Build history of the part. All positions in model axes, mm. Face numbers are marked on the shaded views. A direction names the side the tool comes from. Round coordinates to 2 decimals unless told otherwise and drop trailing zeros. Write each loop counter-clockwise with the first axis right and the second up, starting at its lowest first coordinate (ties: lowest second). Pieces come first, ordered by that corner, then holes.
from build123d import *

# Parameters (mm, degrees)
SKETCH2_R           = 1.315325132
SKETCH2_R_2         = 1.3
BOSS_EXTRUDE1_DEPTH = 3
CUT_EXTRUDE1_DEPTH  = 10
BOSS_EXTRUDE3_DEPTH = 15
SKETCH6_R           = 2.2
CUT_EXTRUDE2_DEPTH  = 10


with BuildPart() as part:
    # Sketch2 → Boss-Extrude1 (new body)
    with BuildSketch(Plane.XZ):
        with BuildLine():
            Line((-23.009319596, 31.276283835), (22.990680404, 31.490636875))
            ThreePointArc((22.990680404, 31.490636875), (24.41091474, 30.908163296), (25, 29.490658589))
            Line((25, 29.490658589), (25, -4.5))
            ThreePointArc((25, -4.5), (25.585786438, -5.914213562), (27, -6.5))
            Line((27, -6.5), (38, -6.5))
            ThreePointArc((38, -6.5), (39.414213562, -7.085786438), (40, -8.5))
            Line((40, -8.5), (40, -34.5))
            ThreePointArc((40, -34.5), (39.414213562, -35.914213562), (38, -36.5))
            Line((38, -36.5), (-38, -36.5))
            ThreePointArc((-38, -36.5), (-39.414213562, -35.914213562), (-40, -34.5))
            Line((-40, -34.5), (-40, -8.5))
            ThreePointArc((-40, -8.5), (-39.414213562, -7.085786438), (-38, -6.5))
            Line((-38, -6.5), (-27, -6.5))
            ThreePointArc((-27, -6.5), (-25.585786438, -5.914213562), (-25, -4.5))
            Line((-25, -4.5), (-25, 29.276305549))
            ThreePointArc((-25, 29.276305549), (-24.417504708, 30.687220289), (-23.009319596, 31.276283835))
        make_face()
        with Locations(Location((22.009080877, 28.712344932, 0), (0, 0, 270))):
            Circle(SKETCH2_R, mode=Mode.SUBTRACT)
        with Locations(Location((-22, 28.7, 0), (0, 0, 270))):
            Circle(SKETCH2_R_2, mode=Mode.SUBTRACT)
        with Locations(Location((-33.75, -27.3, 0), (0, 0, 270))):
            Circle(SKETCH2_R_2, mode=Mode.SUBTRACT)
        with Locations(Location((33.75, -27.3, 0), (0, 0, 270))):
            Circle(SKETCH2_R_2, mode=Mode.SUBTRACT)
    extrude(amount=BOSS_EXTRUDE1_DEPTH)

    # Sketch3 → Cut-Extrude1 (cut)
    with BuildSketch(Plane.XZ.offset(3)):
        with BuildLine():
            Line((-18, 26.233664787), (18, 26.233664787))
            ThreePointArc((18, 26.233664787), (19.414213562, 25.64787835), (20, 24.233664787))
            Line((20, 24.233664787), (20, -14.643421245))
            ThreePointArc((20, -14.643421245), (19.414213562, -16.057634807), (18, -16.643421245))
            Line((18, -16.643421245), (-18, -16.643421245))
            ThreePointArc((-18, -16.643421245), (-19.414213562, -16.057634807), (-20, -14.643421245))
            Line((-20, -14.643421245), (-20, 24.233664787))
            ThreePointArc((-20, 24.233664787), (-19.414213562, 25.64787835), (-18, 26.233664787))
        make_face()
    extrude(amount=-CUT_EXTRUDE1_DEPTH, mode=Mode.SUBTRACT)

    # Sketch5 → Boss-Extrude3 (add)
    with BuildSketch(Plane.XZ.offset(3)):
        with BuildLine():
            Line((-40, -32.5), (40, -32.5))
            Line((40, -32.5), (40, -34.5))
            ThreePointArc((40, -34.5), (39.414213562, -35.914213562), (38, -36.5))
            Line((38, -36.5), (-38, -36.5))
            ThreePointArc((-38, -36.5), (-39.414213562, -35.914213562), (-40, -34.5))
            Line((-40, -34.5), (-40, -32.5))
        make_face()
    extrude(amount=BOSS_EXTRUDE3_DEPTH)

    # Sketch6 → Cut-Extrude2 (cut)
    with BuildSketch(Plane.XY.offset(-32.5)):
        with Locations((-25, -10.5)):
            Circle(SKETCH6_R)
        with Locations((25, -10.5)):
            Circle(SKETCH6_R)
    extrude(amount=-CUT_EXTRUDE2_DEPTH, mode=Mode.SUBTRACT)


solid = part.part
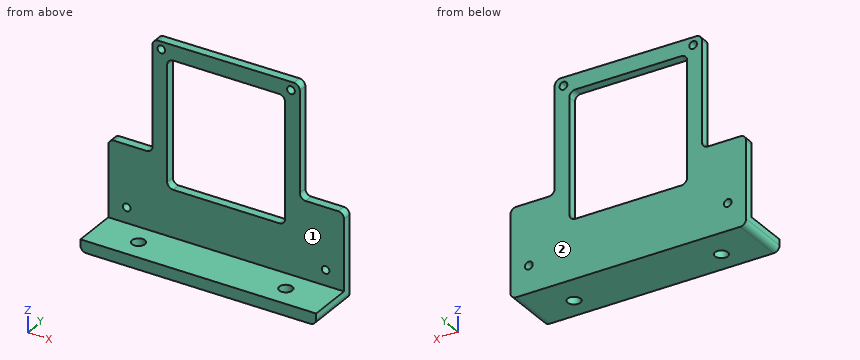
1) Pin check, flat tips, straight feed: pin 1 Ø3 at (x, z) = (-22, 28.7) entering from -Y; pin 2 Ø1.5 at (x, y) = (-31.5, -13) entering from +Z; pin 3 Ø2.5 at (x, y) = (-34, -2) entering from +Z. Stop position of each tip, or through.
Results:
pin 1: stops at y = -3
pin 2: stops at z = -32.5
pin 3: stops at z = -6.5
2) Wall check: L1, parallel to X at y = -1.15, z = -27.3; L2, parallel to X at y = -1, z = 28.7; L3, parallel to Y at x = 25, z = -35.4. Give the ranges that are in metal, low to high.
Results:
L1: x = -40 to -35.05, -32.45 to 32.45, 35.05 to 40
L2: x = -25 to -23.3, -20.7 to 20.69, 23.32 to 25
L3: y = -18 to -12.7, -8.3 to 0
3) Which spindle directions (+Z, -Z, +X, -X, +Y, -Y) get a long thin tool onto all of the face, cutting with end or side? Do the marked faces 1 and 2. Say none if no direction does.
Results:
face 1: +Z, +X, -X, -Y
face 2: +Z, -Z, +X, -X, +Y
4) Slice it at B-B (x = 33.75). Write the cut outline in (y, z).
Results:
outline: (-18, -36.5) - (0, -36.5) - (0, -28.6) - (-3, -28.6) - (-3, -32.5) - (-18, -32.5) - close; (-3, -26) - (0, -26) - (0, -6.5) - (-3, -6.5) - close
5) Slice it at C-C (y = -14.75). Write the cut outline in (x, z), plus the area to 3 significant figures.
Results:
outline: (-40, -34.5) arc R2 ccw to (-38, -36.5) - (38, -36.5) arc R2 ccw to (40, -34.5) - (40, -32.5) - (-40, -32.5) - close
area: 318 mm2
6) Slice it at D-D (x = -5). Write the cut outline in (y, z), plus the area to 3 significant figures.
Results:
outline: (-18, -36.5) - (0, -36.5) - (0, -16.64) - (-3, -16.64) - (-3, -32.5) - (-18, -32.5) - close; (-3, 26.23) - (0, 26.23) - (0, 31.36) - (-3, 31.36) - close
area: 135 mm2
7) Slice it at A-A (z = -27.3). Write the cut outline in (x, y).
Results:
outline: (-40, -3) - (-35.05, -3) - (-35.05, 0) - (-40, 0) - close; (-32.45, -3) - (32.45, -3) - (32.45, 0) - (-32.45, 0) - close; (35.05, -3) - (40, -3) - (40, 0) - (35.05, 0) - close
